Part model, mm, in its own coordinate system. A direction names the side the tool comes from. Give positions to 0.01 mm unless a question says otherwise; leave off trailing zeros. Write each loop counter-clockwise with the first axis right and the second up, starting at its lowest first coordinate (ties: lowest second). Pieces come first, ordered by that corner, then holes. Notation, with made-up numbers: M 6,14 L 54,14 A29 cw 54,51 Z; hole C 69,43.25 d3. An arc over 180 degrees is marked long. Use CSV: the item, a comma, the result in double quotes. Start each with the question number.
Item 1: Cut at C-C (z = 7.5). List the corners of the cut face in (x, y) (3 decimals), then the cut area to 3 significant figures.
Item 2: Cut at B-B (x = 35.5). List the corners of the cut face in (y, z).
Item 3: Which spindle directions (+Z, -Z, +X, -X, +Y, -Y) get a long thin tool onto all of the face, cutting with end or side? Do faces 1 (the flat face through (28, -6.35, 22)), 2 (the flat face through (22, -16, 6.35)), 3 (the flat face through (12, -15, 12.7)), 4 (the flat face through (7, -25.4, 8)). Say none if no direction does.
Item 4: Cut at D-D (x = 29.5). List the corners of the cut face in (y, z), then the cut area to 3 significant figures.
Item 5: Cut at A-A (y = -13). List the corners of the cut face in (x, z), then the cut area to 3 significant figures.
Item 6: Pin check, flat tips, straight feed: pin 1 (15 mm diameter, centred on x = 5.5, y = -9, fed in from +Z); pin 2 (10 mm diameter, centred on x = 22, z = 21, fed in from +Y); pin 3 (5 mm diameter, centred on x = 31, z = 23.5, fed in from -Y); pin 4 (2 mm diameter, centred on x = 15.5, y = -6, fed in from -Z). Stop position of each tip, or through.
Item 7: Mould opens along X. For faces 5 (the flat face through (28, -3, 25.4)), 6 (the flat face through (0, -13, 6)), 7 (the cylindrical face through (28.775, -16.269, 12.789)) say: released by +X, released by -X, zero draft, split by the parting line, or undercut.
Item 8: Drill centre lines: line 1 (X direction, y = -27, z = 19); line 2 (Z direction, x = 29.5, y = -3); line 3 (Z direction, x = 7.5, y = -15). Where is each one in solid material? Low to high. Write a range as [from, to].
from build123d import *

# Parameters (mm, degrees)
F1_DEPTH = 31.75
F3_DEPTH = 6.35
F4_W     = 19.05
F4_H     = 6.35
F5_DEPTH = 6.35
F4_R     = 3.175
F6_DEPTH = 19.051


with BuildPart() as f1:
    # F0 (on Front) → F1 (new body)
    with BuildSketch(Plane.XZ):
        Polygon((0, 12.7), (0, 0), (6.35, 0), (6.35, 6.35), (38.1, 6.35), (38.1, 19.05), (19.05, 19.05), (19.05, 12.7), align=None)
    extrude(amount=F1_DEPTH)

    # F2 (on face) → F3 (cut)
    with BuildSketch(Plane.XZ.offset(31.75)):
        Polygon((19.05, 6.35), (19.05, 12.7), (0, 12.7), (0, 0), (6.35, 0), (6.35, 6.35), align=None)
    extrude(amount=-F3_DEPTH, mode=Mode.SUBTRACT)

    # F4 (on face) → F5 (join)
    with BuildSketch(Plane.XY.offset(19.05)):
        with Locations((28.575, -3.175)):
            Rectangle(F4_W, F4_H)
    extrude(amount=F5_DEPTH)

    # F4 (on face) → F6 (cut, through all)
    with BuildSketch(Plane.XY.offset(19.05)):
        with Locations((31.115, -18.415)):
            Circle(F4_R)
        with Locations((9.525, -12.065)):
            Circle(F4_R)
    extrude(amount=-F6_DEPTH, mode=Mode.SUBTRACT)


solid = f1.part
Worked answers:
1,outline,"M 0,-25.4 L 19.05,-25.4 L 19.05,-31.75 L 38.1,-31.75 L 38.1,0 L 0,0 Z; hole C 9.525,-12.065 d6.35; hole C 31.115,-18.415 d6.35"
1,area,"1,030 mm^2"
2,outline,"M -31.75,6.35 L 0,6.35 L 0,25.4 L -6.35,25.4 L -6.35,19.05 L -31.75,19.05 Z"
3,face 1,"+Z, +X, -X, -Y"
3,face 2,"-Z, +X, +Y, -Y"
3,face 3,"+Z, -X, +Y, -Y"
3,face 4,"+Z, -Z, -X, -Y"
4,outline,"M -31.75,6.35 L -21.15,6.35 L -21.15,19.05 L -31.75,19.05 Z; M -15.68,6.35 L 0,6.35 L 0,25.4 L -6.35,25.4 L -6.35,19.05 L -15.68,19.05 Z"
4,area,"374 mm^2"
5,outline,"M 0,0 L 6.35,0 L 6.35,6.35 L 6.49,6.35 L 6.49,12.7 L 0,12.7 Z; M 12.56,6.35 L 38.1,6.35 L 38.1,19.05 L 19.05,19.05 L 19.05,12.7 L 12.56,12.7 Z"
5,area,"365 mm^2"
6,pin 1,"stops at z = 12.7"
6,pin 2,"stops at y = 0"
6,pin 3,"stops at y = -6.35"
6,pin 4,"stops at z = 6.35"
7,face 5,"zero draft"
7,face 6,"released by -X"
7,face 7,"undercut"
8,line 1,"x = [19.05, 38.1]"
8,line 2,"z = [6.35, 25.4]"
8,line 3,"z = [6.35, 12.7]"
